```python
from build123d import *

# Parameters (mm, degrees)
F0_W     = 76.2
F0_H     = 203.2
F1_DEPTH = 63.5
F2_W     = 57.8507818282
F2_H     = 49.3930634111
F3_DEPTH = 101.6
F4_R     = 8.255
F5_R     = 8.3312
F6_R     = 5.08
F7_W     = 164.5440448
F7_H     = 76.2
F8_DEPTH = 63.5
F9_R     = 5.08


with BuildPart() as f1:
    # F0 (on Front) → F1 (new body)
    with BuildSketch(Plane.XZ):
        Rectangle(F0_W, F0_H)
    extrude(amount=F1_DEPTH)

    # F2 (on face) → F3 (join)
    with BuildSketch(Plane(origin=(0, 0, -101.6), x_dir=(1, 0, 0), z_dir=(0, 0, -1))):
        with Locations((0, 29.4664166868)):
            Rectangle(F2_W, F2_H)
    extrude(amount=F3_DEPTH)

    # F4
    f4_edges = [f1.edges().sort_by_distance(p)[0] for p in [
        (-28.925391, -54.162948, -152.4),
    ]]
    fillet(f4_edges, radius=F4_R)

    # F5
    f5_edges = [f1.edges().sort_by_distance(p)[0] for p in [
        (28.925391, -54.162948, -152.4),
        (28.925391, -4.769885, -152.4),
        (-28.925391, -4.769885, -152.4),
    ]]
    fillet(f5_edges, radius=F5_R)

    # F6
    f6_edges = [f1.edges().sort_by_distance(p)[0] for p in [
        (28.925391, -29.466417, -203.2),
        (26.485239, -51.722796, -203.2),
        (26.485239, -7.210037, -203.2),
        (0, -4.769885, -203.2),
        (-0.0381, -54.162948, -203.2),
        (-26.507557, -51.745115, -203.2),
        (-28.925391, -29.504517, -203.2),
        (-26.485239, -7.210037, -203.2),
    ]]
    fillet(f6_edges, radius=F6_R)

    # F7 (on face) → F8 (join)
    with BuildSketch(Plane.XZ.offset(63.5)):
        with Locations((0, 63.5)):
            Rectangle(F7_W, F7_H)
    extrude(amount=-F8_DEPTH)

    # F9
    f9_edges = [f1.edges().sort_by_distance(p)[0] for p in [
        (0, -63.5, 101.6),
        (0, 0, 101.6),
        (-60.186011, 0, 25.4),
        (60.186011, 0, 25.4),
        (-60.186011, -63.5, 25.4),
        (60.186011, -63.5, 25.4),
        (82.272022, -31.75, 25.4),
        (82.272022, -31.75, 101.6),
        (82.272022, -63.5, 63.5),
        (82.272022, 0, 63.5),
        (-82.272022, -31.75, 101.6),
        (-82.272022, -31.75, 25.4),
        (-82.272022, -63.5, 63.5),
        (-82.272022, 0, 63.5),
        (-38.1, -63.5, -38.1),
        (38.1, -63.5, -38.1),
        (-38.1, 0, -38.1),
        (38.1, 0, -38.1),
    ]]
    fillet(f9_edges, radius=F9_R)


solid = f1.part
```
Can you work these out from the model? Positions are in its coordinate system, mm. A direction names the side the tool comes from. Give positions to 0.01 mm unless a question says otherwise; leave off trailing zeros. Write each loop counter-clockwise with the first axis right and the second up, starting at its lowest first coordinate (ties: lowest second). Pieces come first, ordered by that corner, then holes. Notation, with made-up numbers: (67.5, 77) - (118.5, 77) arc R27 cw to (118.5, 98) - close; hole circle Ø6 at (15, 37). An arc over 180 degrees is marked (long way). Write item = value, one per line. Start each with the question number.
1. Imagine slicing it at B-B (y = -40). Please give me the cut outline in (x, z), and give its area (3 significant figures).
2. On a 3-axis mill with a long thin cutter (end or side, diameter ignored), from which of +Z, -Z, +X, -X, +Y, -Y can I reach the whole of each face in a straight line? I mean faces 1 (the face through (-28.925, -29, -149)), 2 (the face through (-1, -60, -101.6)), 3 (the face through (57, -32, 25.4)), 4 (the face through (26.42, -7.146, -150.536)). Say none if no direction works.
3. Please list where these lines run through material, in increasing order: line 1 (Z direction, x = 34, y = -35.5); line 2 (Z direction, x = 55, y = -25); line 3 (X direction, y = -31, z = -83).
4. Imagine slicing it at A-A (z = -88). Please give me the cut outline in (x, y).
5. Imagine slicing it at D-D (x = 9). Please give me the cut outline in (y, z).
6. Imagine slicing it at C-C (x = -48). Please give me the cut outline in (y, z), and give its area (3 significant figures).
7. For pin 1 (19.5 mm diameter, centred on x = -64, y = -21, fed in from -Z); pin 2 (1 mm diameter, centred on x = -18.5, z = -170, fed in from -Y); pin 3 (6 mm diameter, centred on y = -20, z = -142, fed in from +X), each with a flat end and sliding along its axis, tell me the tip position at first contact or that it passes through.
Worked answers:
q1.outline = (-82.27, 30.48) arc R5.08 ccw to (-77.19, 25.4) - (-38.1, 25.4) - (-38.1, -101.6) - (-28.93, -101.6) - (-28.93, -198.12) arc R5.08 ccw to (-23.85, -203.2) - (23.85, -203.2) arc R5.08 ccw to (28.93, -198.12) - (28.93, -101.6) - (38.1, -101.6) - (38.1, 25.4) - (77.19, 25.4) arc R5.08 ccw to (82.27, 30.48) - (82.27, 96.52) arc R5.08 ccw to (77.19, 101.6) - (-77.19, 101.6) arc R5.08 ccw to (-82.27, 96.52) - close
q1.area = 28,100 mm2
q2.face_1 = -Z, -X, +Y, -Y
q2.face_2 = -Z
q2.face_3 = -Z, +X, +Y, -Y
q2.face_4 = -Z, +X, +Y
q3.line_1 = -101.6 to 101.6
q3.line_2 = 25.4 to 101.6
q3.line_3 = -38.1 to 38.1
q4.outline = (-38.1, -58.42) arc R5.08 ccw to (-33.02, -63.5) - (33.02, -63.5) arc R5.08 ccw to (38.1, -58.42) - (38.1, -5.08) arc R5.08 ccw to (33.02, 0) - (-33.02, 0) arc R5.08 ccw to (-38.1, -5.08) - close
q5.outline = (-63.5, -101.6) - (-54.16, -101.6) - (-54.16, -198.12) arc R5.08 ccw to (-49.08, -203.2) - (-9.85, -203.2) arc R5.08 ccw to (-4.77, -198.12) - (-4.77, -101.6) - (0, -101.6) - (0, 96.52) arc R5.08 ccw to (-5.08, 101.6) - (-58.42, 101.6) arc R5.08 ccw to (-63.5, 96.52) - close
q6.outline = (-63.5, 30.48) arc R5.08 ccw to (-58.42, 25.4) - (-5.08, 25.4) arc R5.08 ccw to (0, 30.48) - (0, 96.52) arc R5.08 ccw to (-5.08, 101.6) - (-58.42, 101.6) arc R5.08 ccw to (-63.5, 96.52) - close
q6.area = 4,820 mm2
q7.pin_1 = 25.4
q7.pin_2 = -54.16
q7.pin_3 = 28.93
